Part model, mm, in its own coordinate system. A direction names the side the tool comes from. Round coordinates to 2 decimals unless told otherwise and drop trailing zeros. Order: outer loops, then holes, each group sorted by start corner. A loop starts at its lowest first (then second) coordinate and runs counter-clockwise, first axis right, second up. Notation, with made-up numbers: M 74,80 L 101,80 A18 cw 101,100 Z; hole C 76.5,4.25 d11. An arc over 180 degrees is marked long. One line per question, with ' | ' between items.
from build123d import *

# Parameters (mm, degrees)
SKETCH002_W     = 97
SKETCH002_H     = 39.7
PAD002_DEPTH    = 9.2
SKETCH003_W     = 95.6
SKETCH003_H     = 38.3
POCKET_DEPTH    = 8.2
POCKET001_DEPTH = 97.001
SKETCH005_W     = 32.5
SKETCH005_H     = 6
SKETCH005_W_2   = 26.2
SKETCH005_W_3   = 5
POCKET002_DEPTH = 3.701
POCKET003_DEPTH = 32.701
POCKET004_DEPTH = 0.5
SKETCH008_W     = 9.8
SKETCH008_H     = 5
POCKET005_DEPTH = 2


with BuildPart() as part:
    # Sketch002 → Pad002 (new body)
    with BuildSketch(Plane.XY):
        Rectangle(SKETCH002_W, SKETCH002_H)
    extrude(amount=PAD002_DEPTH)

    # Sketch003 (on Face5 of Pad002) → Pocket (cut)
    with BuildSketch(Plane(origin=(0, 0, 0), x_dir=(1, 0, 0), z_dir=(0, 0, -1))):
        Rectangle(SKETCH003_W, SKETCH003_H)
    extrude(amount=-POCKET_DEPTH, mode=Mode.SUBTRACT)

    # Sketch004 (on Face3 of Pocket) → Pocket001 (cut, through all)
    with BuildSketch(Plane.YZ.offset(48.5)):
        Polygon((19.15, 5.5), (-19.15, 5.5), (-19.15, 0), (-19.15, -1), (19.15, -1), (19.15, 0), align=None)
    extrude(amount=-POCKET001_DEPTH, mode=Mode.SUBTRACT)

    # Sketch005 (on Face8 of Pocket001) → Pocket002 (cut, through all)
    with BuildSketch(Plane(origin=(0, 0, 5.5), x_dir=(1, 0, 0), z_dir=(0, 0, -1))):
        with Locations((0, 15.85)):
            Rectangle(SKETCH005_W, SKETCH005_H)
        with Locations((-31.35, 15.85)):
            Rectangle(SKETCH005_W_2, SKETCH005_H)
        with Locations((-48.95, 15.85)):
            Rectangle(SKETCH005_W_3, SKETCH005_H)
        with Locations((31.35, 15.85)):
            Rectangle(SKETCH005_W_2, SKETCH005_H)
        with Locations((48.95, 15.85)):
            Rectangle(SKETCH005_W_3, SKETCH005_H)
    extrude(amount=-POCKET002_DEPTH, mode=Mode.SUBTRACT)

    # Sketch006 (on Face20 of Pocket002) → Pocket003 (cut, through all)
    with BuildSketch(Plane.XZ.offset(12.85)):
        with BuildLine():
            Line((-37, 13.1), (37, 13.1))
            ThreePointArc((38, 12.1), (37.707107, 12.807107), (37, 13.1))
            Line((38, 12.1), (38, -12.1))
            ThreePointArc((37, -13.1), (37.707107, -12.807107), (38, -12.1))
            Line((37, -13.1), (-37, -13.1))
            ThreePointArc((-38, -12.1), (-37.707107, -12.807107), (-37, -13.1))
            Line((-38, -12.1), (-38, 12.1))
            ThreePointArc((-37, 13.1), (-37.707107, 12.807107), (-38, 12.1))
        make_face()
    extrude(amount=-POCKET003_DEPTH, mode=Mode.SUBTRACT)

    # Sketch007 (on Face20 of Pocket003) → Pocket004 (cut)
    with BuildSketch(Plane.YZ.offset(48.5)):
        with BuildLine():
            ThreePointArc((-43.699994, 7.4), (-44.1, 7.000001), (-43.699996, 6.6))
            Line((-43.699996, 6.6), (43.7, 6.6))
            ThreePointArc((43.7, 6.6), (44.1, 7), (43.699999, 7.4))
            Line((-43.699994, 7.4), (43.699999, 7.4))
        make_face()
        with BuildLine():
            ThreePointArc((-43.7, -6.6), (-44.1, -7), (-43.7, -7.4))
            Line((-43.7, -7.4), (43.7, -7.4))
            ThreePointArc((43.7, -7.4), (44.1, -7), (43.7, -6.6))
            Line((-43.7, -6.6), (43.7, -6.6))
        make_face()
    extrude(amount=-POCKET004_DEPTH, mode=Mode.SUBTRACT)

    # Sketch008 (on Face21 of Pocket004) → Pocket005 (cut)
    with BuildSketch(Plane(origin=(0, 19.85, 0), x_dir=(-1, 0, 0), z_dir=(0, 1, 0))):
        with Locations((0, 5)):
            Rectangle(SKETCH008_W, SKETCH008_H)
    extrude(amount=-POCKET005_DEPTH, mode=Mode.SUBTRACT)


solid = part.part
1) Saw through at D-D (x = -4). List the corners of the cut face in (y, z), plus the area to 3 significant figures.
The answers:
outline: M -19.85,0 L -19.15,0 L -19.15,8.2 L -18.85,8.2 L -18.85,9.2 L -19.85,9.2 Z | area: 6.74 mm²
2) Saw through at C-C (z = 2.5). List the corners of the cut face in (x, y), plus the area to 3 significant figures.
The answers:
outline: M -48.5,-19.85 L 48.5,-19.85 L 48.5,-19.15 L -48.5,-19.15 Z; M -48.5,19.15 L -38,19.15 L -38,19.85 L -48.5,19.85 Z; M 38,19.15 L 48.5,19.15 L 48.5,19.85 L 38,19.85 Z | area: 82.6 mm²
3) Probe line 1 (X direction, y = 6.5, z = 7.75); line 2 (Y direction, x = -38.5, z = 0.5); line 3 (X direction, y = 3, z = 8.5). List the from-to ranges inside material, lowest first. Write a range as [from, to].
The answers:
line 1: x = [-48.5, -47.8], [47.8, 48.5] | line 2: y = [-19.85, -19.15], [19.15, 19.85] | line 3: x = [-48.5, -38], [38, 48.5]
4) Two-plate mould, pull along X, no slides. Class faces 6 (the face through (-0.23, -19.02, 9.2)), 7 (the face through (48.5, 3, 8)), 8 (the face through (47.8, 3, 7)), 9 (the face through (-43, 19.15, 4)): released by +X, released by -X, zero draft, split by the parting line, or undercut.
The answers:
face 6: zero draft | face 7: released by +X | face 8: undercut | face 9: undercut
5) Drop flat-ended pins along their axis: pin 1 (5 mm diameter, centred on x = -12.5, z = 1.5, fed in from +Y); pin 2 (1.1 mm diameter, centred on y = -16, z = 8.5, fed in from -X); pin 3 (1.5 mm diameter, centred on y = 11.5, z = 3.5, fed in from +X); pin 4 (0.5 mm diameter, centred on x = 17, z = 9, fed in from +Y). Give the stop position or say it passes through.
The answers:
pin 1: stops at y = -19.15 | pin 2: stops at x = -46.45 | pin 3: passes through | pin 4: stops at y = -12.85
6) Which spindle directions (+Z, -Z, +X, -X, +Y, -Y) get a long thin tool onto all of the face, cutting with end or side? Do faces 1 (the face through (-38, 7, 9)), 2 (the face through (-48, -18.85, 8)), 3 (the face through (48, -18.85, 8)), 4 (the face through (-43, 19.85, 5)), 5 (the face through (43, 19.15, 4)). Say none if no direction does.
The answers:
face 1: +Z, -Z, +Y | face 2: +Z, -Z, -X | face 3: +Z, -Z, +X | face 4: +Z, -Z, +X, -X, +Y | face 5: -Z
7) Saw through at B-B (y = -6). List the corners of the cut face in (x, z).
The answers:
outline: M -48.5,5.5 L -47.8,5.5 L -47.8,8.2 L -38,8.2 L -38,9.2 L -48.5,9.2 Z; M 38,8.2 L 47.8,8.2 L 47.8,5.5 L 48.5,5.5 L 48.5,6.6 L 48,6.6 L 48,7.4 L 48.5,7.4 L 48.5,9.2 L 38,9.2 Z
8) Saw through at A-A (x = 41.5). List the corners of the cut face in (y, z).
The answers:
outline: M -19.85,0 L -19.15,0 L -19.15,8.2 L -18.85,8.2 L -18.85,9.2 L -19.85,9.2 Z; M -12.85,8.2 L 19.15,8.2 L 19.15,0 L 19.85,0 L 19.85,9.2 L -12.85,9.2 Z
